from build123d import *

# Parameters (mm, degrees)
SALIENTE_EXTRUIR1_DEPTH = 3
CROQUIS2_R              = 2.8
CORTAR_EXTRUIR3_DEPTH   = 5.5
CROQUIS3_R              = 5
SALIENTE_EXTRUIR2_DEPTH = 4.1
REDONDEO1_R             = 1


with BuildPart() as part:
    # Croquis1 → Saliente-Extruir1 (new body)
    with BuildSketch(Plane.XY):
        with BuildLine():
            Line((-13.118348224, -13.346885602), (-5.358962429, -8.729934305))
            ThreePointArc((-5.358962429, -8.729934305), (0, -10.243545836), (5.358962429, -8.729934305))
            Line((5.358962429, -8.729934305), (13.118348224, -13.346885602))
            ThreePointArc((13.118348224, -13.346885602), (19.97194541, -11.606711584), (18.231771393, -4.753114398))
            Line((18.231771393, -4.753114398), (10.243545836, 0))
            ThreePointArc((10.243545836, 0), (8.83594818, 5.182301714), (5, 8.94037087))
            Line((5, 8.94037087), (5, 18.2))
            ThreePointArc((5, 18.2), (0, 23.2), (-5, 18.2))
            Line((-5, 18.2), (-5, 8.94037087))
            ThreePointArc((-5, 8.94037087), (-8.83594818, 5.182301714), (-10.243545836, 0))
            Line((-10.243545836, 0), (-18.231771393, -4.753114398))
            ThreePointArc((-18.231771393, -4.753114398), (-19.97194541, -11.606711584), (-13.118348224, -13.346885602))
        make_face()
    extrude(amount=SALIENTE_EXTRUIR1_DEPTH)

    # Croquis2 → Cortar-Extruir3 (cut)
    with BuildSketch(Plane.XY.offset(3)):
        with Locations((0, 18.2)):
            Circle(CROQUIS2_R)
        with Locations((15.675059808, -9.05)):
            Circle(CROQUIS2_R)
        with Locations((-15.675059808, -9.05)):
            Circle(CROQUIS2_R)
    extrude(amount=-CORTAR_EXTRUIR3_DEPTH, mode=Mode.SUBTRACT)

    # Croquis3 → Saliente-Extruir2 (add)
    with BuildSketch(Plane.XY.offset(3)):
        Circle(CROQUIS3_R)
    extrude(amount=SALIENTE_EXTRUIR2_DEPTH)

    # Redondeo1
    redondeo1_edges = [part.edges().sort_by_distance(p)[0] for p in [
        (-5, 0, 3),
    ]]
    fillet(redondeo1_edges, radius=REDONDEO1_R)


solid = part.part
Could you check a few things on this model? Use its own coordinates, in mm. A direction names the side the tool comes from. Give positions to 0.01 mm unless a question says otherwise; leave off trailing zeros. Order: outer loops, then holes, each group sorted by start corner. A loop starts at its lowest first (then second) coordinate and runs counter-clockwise, first axis right, second up.
Item 1: If we section it at D-D, the plane x = 17: Write out the boundary of the cut face in (y, z), plus the area to 3 significant figures.
Item 2: For faces 5 (the face through (5, 14, 1)), 6 (the face through (-1.08, -4.88, 5.53)), 7 (the face through (9.184, -11.006, 1.479)), which set-ups out of +Z, -Z, +X, -X, +Y, -Y let a thin tool reach every point of the face, with its end or its side?
Item 3: If we section it at A-A, the plane x = 0: Write out the boundary of the cut face in (y, z), plus the area to 3 significant figures.
Item 4: I need wall thicknesses on line 1 (X direction, y = -6.5, z = 1.5); line 2 (X direction, y = -11, z = 2.25); line 3 (Y direction, x = 1, z = 2.5). Which ranges of each line are inside material? Lowest first, please.
Item 5: If we mould it in two halves opening along X, with no side actions, what happens to faces 1 (the face through (-5, 14, 1)), 2 (the face through (8.87, 5.12, 1.48)), 3 (the face through (-17.74, -7.16, 1.52)), 4 (the face through (13.61, -7.16, 1.52))? For each: pulls with the +X half, pulls with the -X half, needs draft (parallel to the pull), parting line crosses it, or undercut.
Item 6: If we section it at C-C, the plane y = -11: Write out the boundary of the cut face in (x, z).
Item 7: I'm going to push flat-ended pins straight in: pin 1 (1.5 mm diameter, centred on x = 9.5, y = 7, fed in from -Z); pin 2 (2.5 mm diameter, centred on y = 14, z = 1.5, fed in from +X); pin 3 (3 mm diameter, centred on y = -7, z = 3, fed in from -X); pin 4 (1.5 mm diameter, centred on y = 15.5, z = 1.5, fed in from -X). Where does each tip first touch, or does it pass through?
Item 8: If we section it at B-B, the plane z = 2.25: Write out the boundary of the cut face in (x, y), plus the area to 3 significant figures.
Values:
1. outline: (-13.87, 0) - (-11.52, 0) - (-11.52, 3) - (-13.87, 3) - close; (-6.58, 0) - (-4.02, 0) - (-4.02, 3) - (-6.58, 3) - close
1. area: 14.8 mm2
2. face 5: +Z, -Z, +X, +Y
2. face 6: +Z
2. face 7: +Z, -Z, -Y
3. outline: (-10.24, 0) - (15.4, 0) - (15.4, 3) - (6, 3) arc R1 cw to (5, 4) - (5, 7.1) - (-5, 7.1) - (-5, 4) arc R1 cw to (-6, 3) - (-10.24, 3) - close; (21, 0) - (23.2, 0) - (23.2, 3) - (21, 3) - close
3. area: 125 mm2
4. line 1: x = -19.98 to -16.83, -14.52 to 14.52, 16.83 to 19.98
4. line 2: x = -20.28 to -17.68, -13.67 to -9.17, 9.17 to 13.67, 17.68 to 20.28
4. line 3: y = -10.19 to 15.58, 20.82 to 23.1
5. face 1: pulls with the -X half
5. face 2: pulls with the +X half
5. face 3: undercut
5. face 4: undercut
6. outline: (-20.28, 0) - (-17.68, 0) - (-17.68, 3) - (-20.28, 3) - close; (-13.67, 0) - (-9.17, 0) - (-9.17, 3) - (-13.67, 3) - close; (9.17, 0) - (13.67, 0) - (13.67, 3) - (9.17, 3) - close; (17.68, 0) - (20.28, 0) - (20.28, 3) - (17.68, 3) - close
7. pin 1: passes through
7. pin 2: stops at x = 5
7. pin 3: stops at x = -20.64
7. pin 4: stops at x = -5
8. outline: (-18.23, -4.75) arc R5 ccw to (-13.12, -13.35) - (-5.36, -8.73) arc R10.24 ccw to (5.36, -8.73) - (13.12, -13.35) arc R5 ccw to (18.23, -4.75) - (10.24, 0) arc R10.24 ccw to (5, 8.94) - (5, 18.2) arc R5 ccw to (-5, 18.2) - (-5, 8.94) arc R10.24 ccw to (-10.24, 0) - close; hole circle Ø5.6 at (-15.68, -9.05); hole circle Ø5.6 at (0, 18.2); hole circle Ø5.6 at (15.68, -9.05)
8. area: 623 mm2
